Geometry check sheet. Reference: the model listing, model coordinates, mm. A direction names the side the tool comes from. Coordinates: 2 decimals unless noted, no trailing zeros. Order: outer loops, then holes, each group sorted by start corner. A loop starts at its lowest first (then second) coordinate and runs counter-clockwise, first axis right, second up. Notation, with made-up numbers: (-32, 67) -> (-7, 67) arc R23 ccw to (-7, 79) -> close; hole circle Ø2 at (-40, 25.5). An arc over 180 degrees is marked (long way). Answer as CSV lines item,"result". Start each with the question number.
Autodesk Inventor part; units mm, degrees
ref_plane "YZ Plane" through (0, 0, 0) normal (1, 0, 0) x (0, 1, 0)
ref_plane "XZ Plane" through (0, 0, 0) normal (0, 1, 0) x (-1, 0, 0)
ref_plane "XY Plane" through (0, 0, 0) normal (0, 0, 1) x (1, 0, 0)
sketch "Sketch1" plane through (0, 0, 0) normal (0, 0, 1) x (1, 0, 0)
  arc A0 (20, 100) -> (18.5818, 85) centre (115.8042, 83.3748) ccw
  arc A1 (-53.6995, 210.1948) -> (-40, 203.923) centre (-6.4957, 295.2045) ccw
  line L0 (-10, 117.3205) -> (0, 100)
  line L1 (-40, 169.282) -> (-50, 186.6025)
  line L2 (0, 100) -> (0, 85)
  line L3 (0, 85) -> (18.5818, 85)
  line L4 (-10, 117.3205) -> (-40, 169.282)
  line L5 (-50, 186.6025) -> (-62.9904, 194.1025)
  line L6 (-62.9904, 194.1025) -> (-53.6995, 210.1948)
  line L7 (87.5833, 208.3013) -> (62.5833, 251.6025)
  line L8 (87.5833, 208.3013) -> (112.5833, 165)
  line L9 (-40, 203.923) -> (62.5833, 251.6025)
  line L10 (20, 100) -> (112.5833, 165)
  dimension "d14" = 15
  dimension "d47" = 15
  dimension "d49" = 50
  dimension "d50" = 50
extrude "Extrusion4" add sketch "Sketch1" along normal blind 5.5
fillet "Fillet1" radius 20 2 edges at (112.5833, 165, 2.75) (62.5833, 251.6025, 2.75)
fillet "Fillet2" radius 20 2 edges at (20, 100, 2.75) (-40, 203.923, 2.75)
properties part number "brazos"
Q1. Go/stop test with flat-tipped pins: pin 1 Ø1 at (x, z) = (49.5, 4) entering from -Y; pin 2 Ø2 at (y, z) = (223.5, 3.5) entering from +X; pin 3 Ø1 at (y, z) = (136, 0.5) entering from +X; pin 4 Ø4 at (x, y) = (35, 106) entering from +Z. Record where each tip stops, or that it passes through.
Q2. Release check for a two-part mould opening along X. For faces 1 (the flat face through (-58.41, 202.036, 2.712)), 2 (the cylindrical face through (-51.413, 208.965, 2.712)), 3 (the flat face through (20, 167, 0)), 4 (the flat face through (61.94, 129.445, 2.712)) record: released by +X, released by -X, zero draft, split by the parting line, or undercut.
Q3. Access from +Z, -Z, +X, -X, +Y, -Y to the whole of each face (thin tool, end or side, straight path). Record for faces 5 (the flat face through (0, 93, 3)), 6 (the cylindrical face through (21.4, 98.67, 2.79)).
Q4. Thickness scan on L1, parallel to Y at x = 17.5, z = 1.05; L2, parallel to X at y = 101.5, z = 1.7; L3, parallel to X at y = 108, z = 0.9. Record the ranges inside material, lowest first.
Q5. Sectioned sample at B-B, the plane y = 220.5. Record the cut outline in (x, z), then the cut area to 3 significant figures.
Q6. Sectioned sample at C-C, the plane x = 52. Record the cut outline in (y, z), then the cut area to 3 significant figures.
Q7. Sectioned sample at A-A, the plane z = 4.65. Record the cut outline in (x, y).
Geometry results:
1,pin 1,"stops at y = 120.36"
1,pin 2,"stops at x = 79.39"
1,pin 3,"stops at x = 71.99"
1,pin 4,"passes through"
2,face 1,"released by -X"
2,face 2,"undercut"
2,face 3,"zero draft"
2,face 4,"released by +X"
3,face 5,"+Z, -Z, -X, -Y"
3,face 6,"+Z, -Z, +X, -Y"
4,L1,"y = 85 to 230.65"
4,L2,"x = -0.87 to 23.36"
4,L3,"x = -4.62 to 31.39"
5,outline,"(-4.33, 0) -> (80.54, 0) -> (80.54, 5.5) -> (-4.33, 5.5) -> close"
5,area,"467 mm^2"
6,outline,"(122.47, 0) -> (245.6, 0) -> (245.6, 5.5) -> (122.47, 5.5) -> close"
6,area,"677 mm^2"
7,outline,"(-62.99, 194.1) -> (-50, 186.6) -> (0, 100) -> (0, 85) -> (18.58, 85) arc R97.23 cw to (18.8, 90.12) arc R20 cw to (27.26, 105.1) -> (97.6, 154.48) arc R20 ccw to (103.43, 180.85) -> (87.58, 208.3) -> (71.74, 235.75) arc R20 ccw to (45.98, 243.89) -> (-31.95, 207.66) arc R20 cw to (-49.16, 207.83) arc R97.24 cw to (-53.7, 210.19) -> close"
